Verification items for this drawing (mm, ordinates from the low corner). A direction names the side the tool comes from. Give positions to 0.01 mm unless a question says otherwise; leave off trailing zeros. Loops run counter-clockwise (first coordinate to the right, second up) from the corner with the lowest first, then second, coordinate; pieces in that order, holes last. Notation, with made-up numbers: (17.25, 36) -> (60.25, 36) arc R11 ccw to (60.25, 45) -> close; hole circle Ø2 at (82, -10). An arc over 180 degrees is marked (long way). Answer in a Markdown table with one row per item. Add a question column.
Q1. Set-up check for the marked faces 1 and 2: record each of +Z, -Z, +X, -X, +Y, -Y from which the full face is reachable in a straight line by a thin tool's end or side.
Q2. Section check A-A on y = 8. Enter the section's corners in (x, z), and give its area (3 significant figures).
Q3. Release check for a two-part mould opening along Y. For the marked faces 3, 4 and 5 record: pulls with the +Y half, pulls with the -Y half, needs draft (parallel to the pull), parting line crosses it, or undercut.
Q4. Material ranges on probe 1 along Y at (x, z) = (11, 8); probe 2 along X at (y, z) = (1, 9.5); probe 3 along X at (y, z) = (12.4, 8), recorded low to high.
Q5. Section check C-C on x = 6.5. Enter the section's corners in (y, z).
Q6. Section check B-B on z = 8. Enter the section's corners in (x, y), and give its area (3 significant figures).
Q7. Gauge pin test, flat ends, axial feed: P1, Ø4, axis at x = 8.5, z = 12.5, coming from the -Y side; P2, Ø1, axis at x = 9, y = 3, coming from the -Z side; P3, Ø8, axis at x = 5, z = 11.5, coming from the +Y side. Record the tip position at first contact, or that the pin passes through.
Q8. Section check D-D on y = 13. Enter the section's corners in (x, z) (3 decimals).
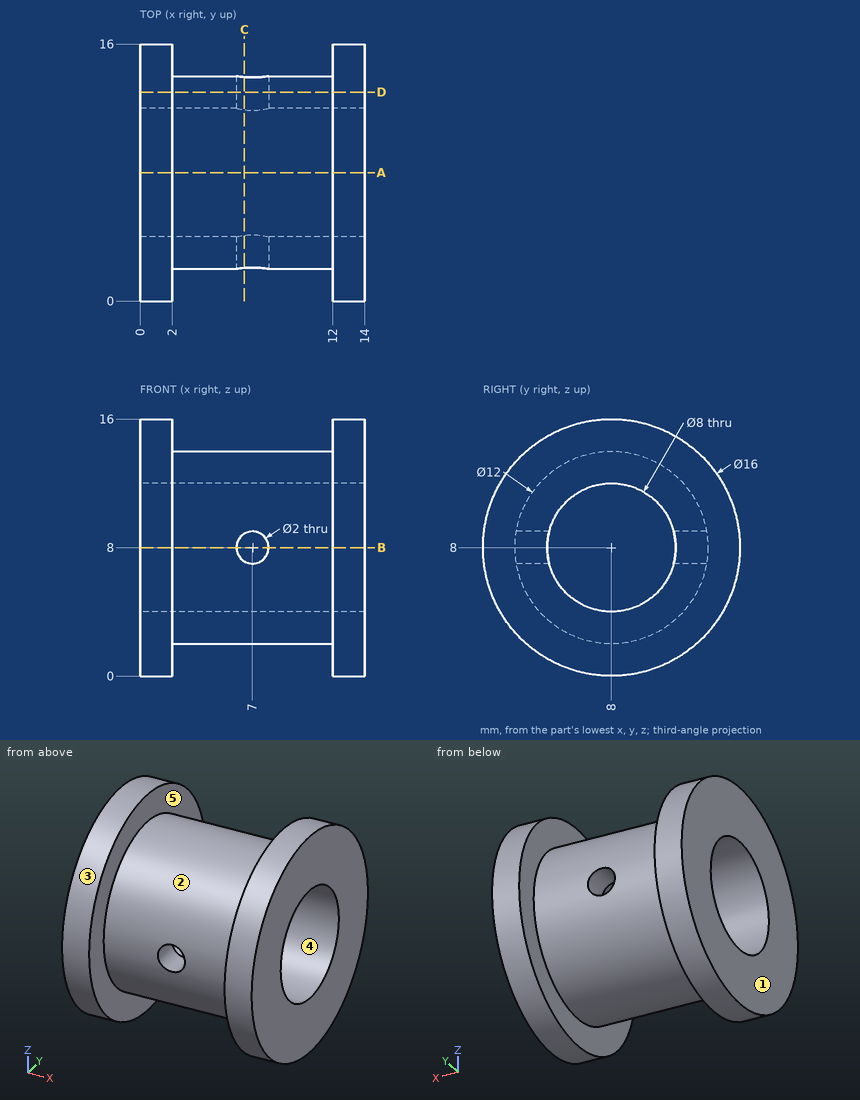
Taken from the geometry:
| question | item | result |
|---|---|---|
| 1 | face 1 | +Z, -Z, -X, +Y, -Y |
| 1 | face 2 | none |
| 2 | outline | (0, 0) -> (2, 0) -> (2, 2) -> (12, 2) -> (12, 0) -> (14, 0) -> (14, 4) -> (0, 4) -> close; (0, 12) -> (14, 12) -> (14, 16) -> (12, 16) -> (12, 14) -> (2, 14) -> (2, 16) -> (0, 16) -> close |
| 2 | area | 72.0 mm² |
| 3 | face 3 | parting line crosses it |
| 3 | face 4 | undercut |
| 3 | face 5 | needs draft |
| 4 | probe 1 | y = 2 to 4, 12 to 14 |
| 4 | probe 2 | x = 0 to 2, 12 to 14 |
| 4 | probe 3 | x = 0 to 6, 8 to 14 |
| 5 | outline | (2.06, 7.13) arc R6 ccw to (13.94, 7.13) -> (11.91, 7.13) arc R4 cw to (4.09, 7.13) -> close; (2.06, 8.87) -> (4.09, 8.87) arc R4 cw to (11.91, 8.87) -> (13.94, 8.87) arc R6 ccw to start |
| 6 | outline | (0, 0) -> (2, 0) -> (2, 2) -> (6, 2) -> (6, 4) -> (0, 4) -> close; (0, 12) -> (6, 12) -> (6, 14) -> (2, 14) -> (2, 16) -> (0, 16) -> close; (8, 2) -> (12, 2) -> (12, 0) -> (14, 0) -> (14, 4) -> (8, 4) -> close; (8, 12) -> (14, 12) -> (14, 16) -> (12, 16) -> (12, 14) -> (8, 14) -> close |
| 6 | area | 64.0 mm² |
| 7 | P1 | stops at y = 2.55 |
| 7 | P2 | stops at z = 4.03 |
| 7 | P3 | stops at y = 15.95 |
| 8 | outline | (0, 1.755) -> (2, 1.755) -> (2, 4.683) -> (12, 4.683) -> (12, 1.755) -> (14, 1.755) -> (14, 14.245) -> (12, 14.245) -> (12, 11.317) -> (2, 11.317) -> (2, 14.245) -> (0, 14.245) -> close; hole circle Ø2 at (7, 8) |
